Geometry check sheet. Reference: the model listing, model coordinates, mm. A direction names the side the tool comes from. Coordinates: 2 decimals unless noted, no trailing zeros. Write each loop counter-clockwise with the first axis right and the second up, starting at its lowest first coordinate (ties: lowest second). Pieces come first, ordered by that corner, then holes. Notation, with made-up numbers: M 34.5,68 L 70.5,68 A27 cw 70.5,99 Z; hole C -17.75,16.25 d10. An arc over 180 degrees is marked long. Write each question's results on one line, items separated by ' | '.
```python
from build123d import *

# Parameters (mm, degrees)
SKETCH2_R           = 2
BOSS_EXTRUDE1_DEPTH = 1.5
SKETCH3_W           = 6
SKETCH3_H           = 4
BOSS_EXTRUDE2_DEPTH = 1


with BuildPart() as part:
    # Sketch2 → Boss-Extrude1 (new body)
    with BuildSketch(Plane.XY):
        with BuildLine():
            Line((-16.5, -19.5), (-6, -19.5))
            ThreePointArc((-6, -19.5), (-5.292893219, -19.792893219), (-5, -20.5))
            Line((-5, -20.5), (-5, -23.5))
            ThreePointArc((-5, -23.5), (-4.707106781, -24.207106781), (-4, -24.5))
            Line((-4, -24.5), (4, -24.5))
            ThreePointArc((4, -24.5), (4.707106781, -24.207106781), (5, -23.5))
            Line((5, -23.5), (5, -20.5))
            ThreePointArc((5, -20.5), (5.292893219, -19.792893219), (6, -19.5))
            Line((6, -19.5), (16.5, -19.5))
            ThreePointArc((16.5, -19.5), (18.621320344, -18.621320344), (19.5, -16.5))
            Line((19.5, -16.5), (19.5, 16.5))
            ThreePointArc((19.5, 16.5), (18.621320344, 18.621320344), (16.5, 19.5))
            Line((16.5, 19.5), (-16.5, 19.5))
            ThreePointArc((-16.5, 19.5), (-18.621320344, 18.621320344), (-19.5, 16.5))
            Line((-19.5, 16.5), (-19.5, -16.5))
            ThreePointArc((-19.5, -16.5), (-18.621320344, -18.621320344), (-16.5, -19.5))
        make_face()
        with Locations((15.25, 15.25)):
            Circle(SKETCH2_R, mode=Mode.SUBTRACT)
        with Locations((15.25, -15.25)):
            Circle(SKETCH2_R, mode=Mode.SUBTRACT)
        with Locations((-15.25, -15.25)):
            Circle(SKETCH2_R, mode=Mode.SUBTRACT)
        with Locations((-15.25, 15.25)):
            Circle(SKETCH2_R, mode=Mode.SUBTRACT)
    extrude(amount=BOSS_EXTRUDE1_DEPTH)

    # Sketch3 → Boss-Extrude2 (add)
    with BuildSketch(Plane.XY.offset(1.5)):
        with Locations((-5, 3.5)):
            Rectangle(SKETCH3_W, SKETCH3_H)
        with Locations((-5, 9.5)):
            Rectangle(SKETCH3_W, SKETCH3_H)
        with Locations((-5, -2.5)):
            Rectangle(SKETCH3_W, SKETCH3_H)
        with Locations((-5, -8.5)):
            Rectangle(SKETCH3_W, SKETCH3_H)
        with Locations((-12.5, 9.5)):
            Rectangle(SKETCH3_W, SKETCH3_H)
        with Locations((-12.5, 3.5)):
            Rectangle(SKETCH3_W, SKETCH3_H)
        with Locations((-12.5, -2.5)):
            Rectangle(SKETCH3_W, SKETCH3_H)
        with Locations((-12.5, -8.5)):
            Rectangle(SKETCH3_W, SKETCH3_H)
        with Locations((12.5, -8.5)):
            Rectangle(SKETCH3_W, SKETCH3_H)
        with Locations((12.5, -2.5)):
            Rectangle(SKETCH3_W, SKETCH3_H)
        with Locations((12.5, 3.5)):
            Rectangle(SKETCH3_W, SKETCH3_H)
        with Locations((12.5, 9.5)):
            Rectangle(SKETCH3_W, SKETCH3_H)
        with Locations((5, -8.5)):
            Rectangle(SKETCH3_W, SKETCH3_H)
        with Locations((5, -2.5)):
            Rectangle(SKETCH3_W, SKETCH3_H)
        with Locations((5, 3.5)):
            Rectangle(SKETCH3_W, SKETCH3_H)
        with Locations((5, 9.5)):
            Rectangle(SKETCH3_W, SKETCH3_H)
        with Locations((8.5, 15.5)):
            Rectangle(SKETCH3_W, SKETCH3_H)
        with Locations((-8.5, 15.5)):
            Rectangle(SKETCH3_W, SKETCH3_H)
        with Locations((8.5, -15.5)):
            Rectangle(SKETCH3_W, SKETCH3_H)
        with Locations((-8.5, -15.5)):
            Rectangle(SKETCH3_W, SKETCH3_H)
    extrude(amount=BOSS_EXTRUDE2_DEPTH)


solid = part.part
```
Q1. Sectioned sample at C-C on x = 10. Record the cut outline in (y, z).
Geometry check:
outline: M -19.5,0 L 19.5,0 L 19.5,1.5 L 17.5,1.5 L 17.5,2.5 L 13.5,2.5 L 13.5,1.5 L 11.5,1.5 L 11.5,2.5 L 7.5,2.5 L 7.5,1.5 L 5.5,1.5 L 5.5,2.5 L 1.5,2.5 L 1.5,1.5 L -0.5,1.5 L -0.5,2.5 L -4.5,2.5 L -4.5,1.5 L -6.5,1.5 L -6.5,2.5 L -10.5,2.5 L -10.5,1.5 L -13.5,1.5 L -13.5,2.5 L -17.5,2.5 L -17.5,1.5 L -19.5,1.5 Z
Q2. Depth check by flat-ended pin: P1, Ø0.5, axis at x = 7, z = 2, coming from the -Y side; P2, Ø0.5, axis at x = 12, z = 2, coming from the +Y side; P3, Ø0.8, axis at y = -22, z = 0.5, coming from the -X side. Enter the tip coordinate at first touch or a pass-through.
Geometry check:
P1: stops at y = -17.5 | P2: stops at y = 11.5 | P3: stops at x = -5
Q3. Access from +Z, -Z, +X, -X, +Y, -Y to the whole of each face (thin tool, end or side, straight path). Record for faces 4 (the flat face through (-11, -19.5, 1)), 5 (the flat face through (12, -2, 2.5)), 6 (the flat face through (-13, -4.5, 2)), 7 (the flat face through (9.5, -9, 2)), 8 (the flat face through (-15.5, 9, 2)).
Geometry check:
face 4: +Z, -Z, -X, -Y | face 5: +Z, +X, -X, +Y, -Y | face 6: +Z, +X, -X | face 7: +Z | face 8: +Z, -X, +Y, -Y
Q4. Mould release check, pull along X, two halves, no side actions. Record for faces 1 (the flat face through (5, 1.5, 2)), 2 (the cylindrical face through (-18.64, -18.6, 0.74)), 3 (the flat face through (2, -3, 2)): pulls with the +X half, pulls with the -X half, needs draft (parallel to the pull), parting line crosses it, or undercut.
Geometry check:
face 1: needs draft | face 2: pulls with the -X half | face 3: undercut
Q5. Sectioned sample at A-A on z = 1.05. Record the cut outline in (x, y).
Geometry check:
outline: M -19.5,-16.5 A3 ccw -16.5,-19.5 L -6,-19.5 A1 cw -5,-20.5 L -5,-23.5 A1 ccw -4,-24.5 L 4,-24.5 A1 ccw 5,-23.5 L 5,-20.5 A1 cw 6,-19.5 L 16.5,-19.5 A3 ccw 19.5,-16.5 L 19.5,16.5 A3 ccw 16.5,19.5 L -16.5,19.5 A3 ccw -19.5,16.5 Z; hole C -15.25,-15.25 d4; hole C -15.25,15.25 d4; hole C 15.25,-15.25 d4; hole C 15.25,15.25 d4
Q6. Sectioned sample at D-D on x = -15. Record the cut outline in (y, z).
Geometry check:
outline: M -19.5,0 L -17.23,0 L -17.23,1.5 L -19.5,1.5 Z; M -13.27,0 L 13.27,0 L 13.27,1.5 L 11.5,1.5 L 11.5,2.5 L 7.5,2.5 L 7.5,1.5 L 5.5,1.5 L 5.5,2.5 L 1.5,2.5 L 1.5,1.5 L -0.5,1.5 L -0.5,2.5 L -4.5,2.5 L -4.5,1.5 L -6.5,1.5 L -6.5,2.5 L -10.5,2.5 L -10.5,1.5 L -13.27,1.5 Z; M 17.23,0 L 19.5,0 L 19.5,1.5 L 17.23,1.5 Z
Q7. Scan lines: probe 1 along Y at (x, z) = (15.25, 0.95); probe 2 along Y at (x, z) = (-5, 1.6); probe 3 along Y at (x, z) = (10, 2.25). Record each from-to range of solid material in increasing order.
Geometry check:
probe 1: y = -19.5 to -17.25, -13.25 to 13.25, 17.25 to 19.5 | probe 2: y = -10.5 to -6.5, -4.5 to -0.5, 1.5 to 5.5, 7.5 to 11.5 | probe 3: y = -17.5 to -13.5, -10.5 to -6.5, -4.5 to -0.5, 1.5 to 5.5, 7.5 to 11.5, 13.5 to 17.5
Q8. Sectioned sample at B-B on y = 15.25. Record the cut outline in (x, z), and give its area (3 significant figures).
Geometry check:
outline: M -19.5,0 L -17.25,0 L -17.25,1.5 L -19.5,1.5 Z; M -13.25,0 L 13.25,0 L 13.25,1.5 L 11.5,1.5 L 11.5,2.5 L 5.5,2.5 L 5.5,1.5 L -5.5,1.5 L -5.5,2.5 L -11.5,2.5 L -11.5,1.5 L -13.25,1.5 Z; M 17.25,0 L 19.5,0 L 19.5,1.5 L 17.25,1.5 Z | area: 58.5 mm2
